Autodesk Inventor part; units mm, degrees
ref_plane "Начальная плоскость" through (0, 0, 0) normal (0, 0, 1) x (1, 0, 0)
ref_plane "Конечная плоскость" through (0, 0, 30) normal (0, 0, 1) x (1, 0, 0)
ref_plane "YZ Plane" through (0, 0, 0) normal (1, 0, 0) x (0, 1, 0)
ref_plane "Начальная плоскость" through (0, 0, 0) normal (0, 0, 1) x (1, 0, 0)
ref_plane "Конечная плоскость" through (0, 0, 30) normal (0, 0, 1) x (1, 0, 0)
sketch "Эскиз" plane through (0, 0, 0) normal (0, 0, 1) x (1, 0, 0)
  line L0 (0, 0) -> (0, 32.5)
  line L1 (0, 32.5) -> (42, 32.5)
  line L2 (42, 32.5) -> (42, 30.3728)
  line L3 (38.319, 26.3855) -> (12.4019, 24.3122)
  line L4 (5.5, 16.836) -> (5.5, 0)
  line L5 (5.5, 0) -> (0, 0) construction
  line L6 (21, 32.5) -> (21, 25) construction
  line L7 (42, 26.68) -> (42, 25) construction
  line L8 (42, 25) -> (21, 25) construction
  line L9 (0, 15) -> (0, -27) construction
  line L10 (-5.539, 0) -> (16.0067, 0) construction
  line L11 (0, 0) -> (0, -32.5)
  line L12 (0, -32.5) -> (42, -32.5)
  line L13 (42, -32.5) -> (42, -30.3728)
  line L14 (38.319, -26.3855) -> (12.4019, -24.3122)
  line L15 (5.5, -16.836) -> (5.5, 0)
  arc A0 (12.4019, 24.3122) -> (5.5, 16.836) centre (13, 16.836) ccw
  arc A1 (5.5, -16.836) -> (12.4019, -24.3122) centre (13, -16.836) ccw
  arc A2 (38.319, 26.3855) -> (42, 30.3728) centre (38, 30.3728) ccw
  arc A3 (42, -30.3728) -> (38.319, -26.3855) centre (38, -30.3728) ccw
  line L16 (0, 35.4) -> (0, -37.4) construction
  line L17 (-11.7637, 0) -> (31.8094, 0) construction
  point P0 (5.5, 23.76)
  point P1 (42, -26.68)
  point P2 (5.5, -23.76)
  point P3 (21, -32.5)
  point P4 (21, -25)
  dimension "d0" = 5.5
  dimension "d1" = 32.5
  dimension "d2" = 42
  dimension "d3" = 7.5
  dimension "d4" = 21
  dimension "d5" = 1.68
  dimension "d23" = 7.5
  dimension "d24" = 4
  dimension "d25" = 0
extrude "Базовый элемент" add sketch "Эскиз" along normal up to surface (30 mm away) from surface at 0
sketch "Sketch3" plane through (0, 0, 0) normal (0, 0, 1) x (1, 0, 0)
  line L0 (0, 0) -> (10, 0)
ref_plane "Work Plane3" through (0, 0, 0) normal (0, -1, 0) x (1, 0, 0)
sketch "Sketch4" plane through (0, 0, 0) normal (0, -1, 0) x (1, 0, 0)
  line L0 (-2, 0) -> (12, 0)
  line L1 (-2, 30) -> (12, 30)
  dimension "d29" = 30
equation "\"d0\" = G_T"
equation "\"d1\" = 0.5 * G_H"
equation "\"d2\" = G_W"
equation "\"d3\" = G_T1"
equation "\"d4\" = G_C"
equation "\"d23\" = G_IR"
equation "\"d24\" = G_ER"
equation "\"d6\" = G_L"
equation "\"G_W\" = 42"
equation "\"G_H\" = 65"
equation "\"G_T\" = 5.5"
equation "\"G_T1\" = 7.5"
equation "\"G_NG\" = 0.08"
equation "\"G_ER\" = 4"
equation "\"G_IR\" = 7.5"
equation "\"G_C\" = 21"
equation "\"G_L\" = d29"
equation "\"ex\" = 0"
equation "\"G_OFFSET_START\" = 0"
equation "\"G_OFFSET_END\" = 0"
properties part number "DIN1026-1 - U 65 - 30" material "Сталь, мягкая"
Input: part model. Units: mm. Frame: model coordinates. A direction names the side the tool comes from. Round coordinates to 2 decimals unless told otherwise and drop trailing zeros. Order: outer loops, then holes, each group sorted by start corner. A loop starts at its lowest first (then second) coordinate and runs counter-clockwise, first axis right, second up. Notation, with made-up numbers: (-11.5, 41.25) - (23.5, 41.25) arc R24 cw to (23.5, 55.25) - close; hole circle Ø11 at (-6, 27.25). An arc over 180 degrees is marked (long way). One line per question, with ' | ' between items. Start each with the question number.
1) Cut plane C-C, the plane x = 39. Return the cut outline in (y, z).
2) Cut plane D-D, the plane y = -11. Return the cut outline in (x, z).
3) Contact query for flat-ended pins moving along their axis: P1, Ø2, axis at y = 17, z = 19, coming from the +X side; P2, Ø5, axis at y = -14, z = 3.5, coming from the +X side; P3, Ø1, axis at y = -12, z = 10.5, coming from the -X side; P4, Ø8, axis at y = -16.5, z = 8, coming from the +X side. Output: stop coordinate, or through.
4) Cut plane A-A, the plane x = 31.5. Return the cut outline in (y, z).
5) Pull-direction query (Y, two-part tool) for faces 1 (the flat face through (5, 3, 30)), 2 (the flat face through (25.542, 25.363, 14.79)), 3 (the flat face through (21, 32.5, 15)); classes: +Y half, -Y half, draft (parallel to the pull), parting line (faces both ways), or undercut.
6) Cut plane B-B, the plane z = 5.5. Return the cut outline in (x, y).
7) Ray query, probe 1 along X at (y, z) = (3.5, 21); probe 2 along Y at (x, z) = (28.5, 24); probe 3 along Y at (x, z) = (33, 18.75). Return the intervals inside material, ascending.
8) Set-up query: faces 4 (the flat face through (21, -32.5, 15)), 5 (the flat face through (25.542, -25.363, 14.79)). Return all of +Z, -Z, +X, -X, +Y, -Y with unobstructed straight access to the full face (end or side cutting, diameter ignored); none if empty.
Worked out:
1) outline: (-32.5, 0) - (-26.5, 0) - (-26.5, 30) - (-32.5, 30) - close; (26.5, 0) - (32.5, 0) - (32.5, 30) - (26.5, 30) - close
2) outline: (0, 0) - (5.5, 0) - (5.5, 30) - (0, 30) - close
3) P1: stops at x = 5.59 | P2: stops at x = 5.5 | P3: stops at x = 0 | P4: stops at x = 6.46
4) outline: (-32.5, 0) - (-25.84, 0) - (-25.84, 30) - (-32.5, 30) - close; (25.84, 0) - (32.5, 0) - (32.5, 30) - (25.84, 30) - close
5) face 1: draft | face 2: undercut | face 3: +Y half
6) outline: (0, -32.5) - (42, -32.5) - (42, -30.37) arc R4 ccw to (38.32, -26.39) - (12.4, -24.31) arc R7.5 cw to (5.5, -16.84) - (5.5, 16.84) arc R7.5 cw to (12.4, 24.31) - (38.32, 26.39) arc R4 ccw to (42, 30.37) - (42, 32.5) - (0, 32.5) - close
7) probe 1: x = 0 to 5.5 | probe 2: y = -32.5 to -25.6, 25.6 to 32.5 | probe 3: y = -32.5 to -25.96, 25.96 to 32.5
8) face 4: +Z, -Z, +X, -X, -Y | face 5: +Z, -Z, +X
